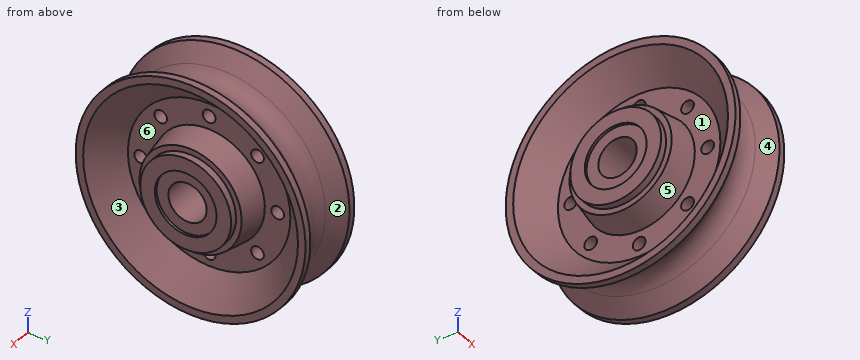
from build123d import *

# Parameters (mm, degrees)
SKETCH3_R          = 1.58676474
CUT_EXTRUDE1_DEPTH = 42.707767281
CIRPATTERN1_COUNT  = 8
SKETCH4_R          = 14.605
SKETCH4_R_2        = 11.303
CUT_EXTRUDE2_DEPTH = 1.719791667
SKETCH5_R          = 7.6835
CUT_EXTRUDE3_DEPTH = 0.635


with BuildPart() as part:
    # Sketch1 → Revolve1 (revolve)
    with BuildSketch(Plane.XY, mode=Mode.PRIVATE) as revolve1_sk:
        with BuildLine():
            Line((6.879166667, 28.575), (8.598958333, 28.575))
            Line((8.598958333, 28.575), (8.598958333, 12.7))
            Line((8.598958333, 12.7), (10.31875, 12.7))
            Line((10.31875, 12.7), (10.31875, 4.7625))
            Line((10.31875, 4.7625), (-10.31875, 4.7625))
            Line((-10.31875, 4.7625), (-10.31875, 12.7))
            Line((-10.31875, 12.7), (-8.598958333, 12.7))
            Line((-8.598958333, 12.7), (-8.598958333, 28.575))
            Line((-8.598958333, 28.575), (-6.879166667, 28.575))
            Line((-6.879166667, 28.575), (-3.359436659, 25.07226429))
            ThreePointArc((-3.359436659, 25.07226429), (0, 23.6855), (3.359436659, 25.07226429))
            Line((3.359436659, 25.07226429), (6.879166667, 28.575))
        make_face()
    revolve(revolve1_sk.sketch.rotate(Axis((-10.31875, 0, 0), (1, 0, 0)), 90), axis=Axis((-10.31875, 0, 0), (1, 0, 0)))

    # Sketch2 → Cut-Revolve1 (revolve, cut)
    with BuildSketch(Plane.XY, mode=Mode.PRIVATE) as cut_revolve1_sk:
        Polygon((-10.31875, 12.7), (-8.598958333, 12.7), (-2.06375, 13.852333554), (-2.06375, 20.199392515), (-10.31875, 28.414534933), align=None)
        Polygon((10.31875, 12.7), (10.31875, 28.414534933), (2.06375, 20.199392515), (2.06375, 13.852333554), (8.598958333, 12.7), align=None)
    revolve(cut_revolve1_sk.sketch.rotate(Axis((-10.31875, 0, 0), (1, 0, 0)), 90), axis=Axis((-10.31875, 0, 0), (1, 0, 0)), mode=Mode.SUBTRACT)

    # Sketch3 → Cut-Extrude1 (cut, symmetric)
    with BuildSketch(Plane(origin=(0, 0, 0), x_dir=(0, 0, -1), z_dir=(1, 0, 0))):
        with Locations((0, 17.025863034)):
            Circle(SKETCH3_R)
    cut_extrude1 = extrude(amount=CUT_EXTRUDE1_DEPTH, both=True, mode=Mode.SUBTRACT)

    # CirPattern1: Cut-Extrude1 ×8 about axis
    cirpattern1_axis = Axis((0, 0, 0), (1, 0, 0))
    for i in range(1, CIRPATTERN1_COUNT):
        add(cut_extrude1.rotate(cirpattern1_axis, i * 360 / CIRPATTERN1_COUNT), mode=Mode.SUBTRACT)

    # Sketch4 → Cut-Extrude2 (cut)
    with BuildSketch(Plane.ZY.offset(10.31875)):
        Circle(SKETCH4_R)
        Circle(SKETCH4_R_2, mode=Mode.SUBTRACT)
    cut_extrude2 = extrude(amount=-CUT_EXTRUDE2_DEPTH, mode=Mode.SUBTRACT)

    # Sketch5 → Cut-Extrude3 (cut)
    with BuildSketch(Plane.ZY.offset(10.31875)):
        Circle(SKETCH5_R)
    cut_extrude3 = extrude(amount=-CUT_EXTRUDE3_DEPTH, mode=Mode.SUBTRACT)

    # Mirror1: Cut-Extrude2, Cut-Extrude3 across plane
    add(cut_extrude2.mirror(Plane(origin=(0, 0, 0), x_dir=(0, 0, 1), z_dir=(1, 0, 0))), mode=Mode.SUBTRACT)
    add(cut_extrude3.mirror(Plane(origin=(0, 0, 0), x_dir=(0, 0, 1), z_dir=(1, 0, 0))), mode=Mode.SUBTRACT)


solid = part.part
Build history of the part. All positions in model axes, mm. Face numbers are marked on the shaded views. A direction names the side the tool comes from. Give positions to 0.01 mm unless a question says otherwise; leave off trailing zeros. Order: outer loops, then holes, each group sorted by start corner. A loop starts at its lowest first (then second) coordinate and runs counter-clockwise, first axis right, second up. Notation, with made-up numbers: M -38.75,-21.75 L -32.75,-21.75 A5 ccw -32.75,-15.75 Z; hole C 58,-25 d8. An arc over 180 degrees is marked long. Use one line per item in the form item = value.
1) Saw through at A-A (z = 0). State how many separate pieces and enclosed holes the cut face has, plus the area to 3 significant figures.
Calculated:
separate_pieces = 4
enclosed_holes = 0
area = 480 mm2
2) Two-plate mould, pull along X, no slides. Class the marked faces 1, 2, 3 and 4: released by +X, released by -X, zero draft, split by the parting line, or undercut.
Calculated:
face_1 = released by -X
face_2 = undercut
face_3 = released by +X
face_4 = undercut
3) Drop flat-ended pins along their axis: pin 1 (1.5 mm diameter, centred on x = -2, z = -11.5, fed in from +Y); pin 2 (5 mm diameter, centred on y = -12.04, z = -12.04, fed in from +X); pin 3 (2 mm diameter, centred on x = 3, z = 21.5, fed in from -Y); pin 4 (1.9 mm diameter, centred on y = 0, z = -17.03, fed in from -X). Give the stop position or say it passes through.
Calculated:
pin_1 = 21.82
pin_2 = 2.06
pin_3 = -14.63
pin_4 = through
4) Probe probe 1 along Z at (x, y) = (-5.5, -9); probe 2 along Y at (x, z) = (-4.5, -12); probe 3 along Z at (x, y) = (-2.5, -3). List the from-to ranges inside material, lowest first.
Calculated:
probe_1 = -25.67 to -21.84, -9.72 to 9.72, 21.84 to 25.67
probe_2 = -23.3 to -19.18, -6.01 to 6.01, 19.18 to 23.3
probe_3 = -24.21 to -20.41, -13.44 to -3.7, 3.7 to 13.44, 20.41 to 24.21
5) Tool access for the marked faces 5 and 6: list every direction of +Z, -Z, +X, -X, +Y, -Y with a clear straight run to the whole face (end or side of a thin tool).
Calculated:
face_5 = -X
face_6 = +X
6) Saw through at C-C (x = -5.5). Give the cut face in (y, z) (1 decimal).
Calculated:
outline = C 0,0 d54.4; C 0,0 d26.5; hole C 0,0 d47.2; hole C 0,0 d9.5
